Could you check a few things on this drawing? It's one solid part, dimensions in mm from its lowest x, y, z. Give positions to 0.01 mm unless a question says otherwise; leave off trailing zeros. Loops run counter-clockwise (first coordinate to the right, second up) from the corner with the lowest first, then second, coordinate; pieces in that order, holes last. Notation, with made-up numbers: (-10.5, 13) -> (18.5, 13) arc R30 cw to (18.5, 44) -> close; hole circle Ø6 at (85.5, 53.5). An arc over 180 degrees is marked (long way). Use CSV: the item, a comma, the result in double quotes.
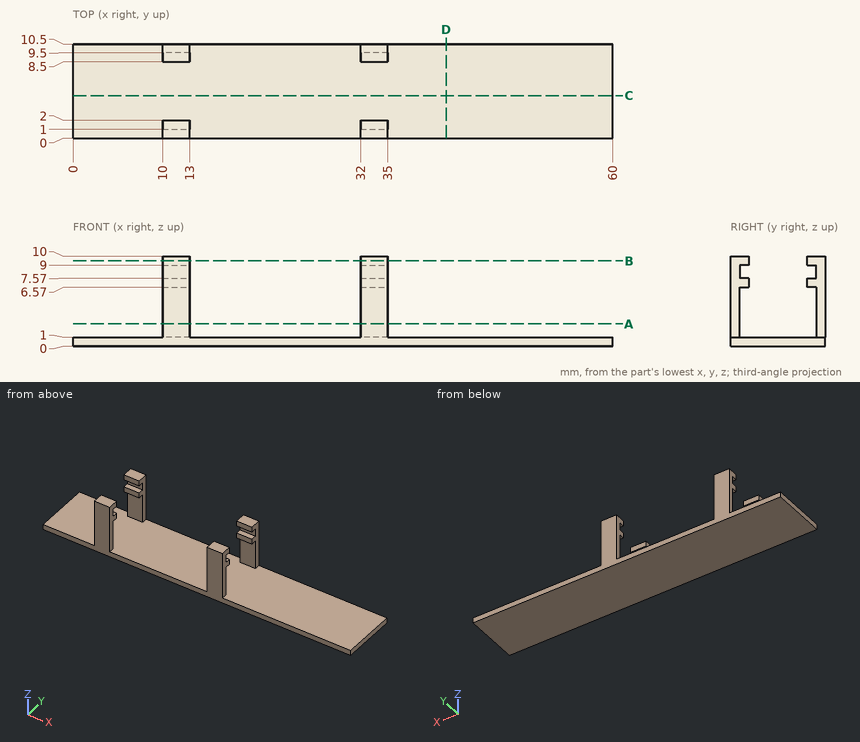
(1) If I drill on L1, parallel to X at y = 9.75, z = 7; L2, parallel to Z at x = 10.5, y = 7.25, over which ranges is the centre line in solid material (lowest first)? Write a range as from..to.
Answer sheet:
L1,"x = 10..13, 32..35"
L2,"z = 0..1"
(2) If we section it at A-A, the plane z = 2.5: Write out the boundary of the cut face in (x, y), then the cut area to 3 significant figures.
Answer sheet:
outline,"(10, 0) -> (13, 0) -> (13, 1) -> (10, 1) -> close; (10, 9.5) -> (13, 9.5) -> (13, 10.5) -> (10, 10.5) -> close; (32, 0) -> (35, 0) -> (35, 1) -> (32, 1) -> close; (32, 9.5) -> (35, 9.5) -> (35, 10.5) -> (32, 10.5) -> close"
area,"12.0 mm2"
(3) If we section it at C-C, the plane y = 4.75: Write out the boundary of the cut face in (x, z).
Answer sheet:
outline,"(0, 0) -> (60, 0) -> (60, 1) -> (0, 1) -> close"
(4) If we section it at B-B, the plane z = 9.5: Write out the boundary of the cut face in (x, y), then the cut area to 3 significant figures.
Answer sheet:
outline,"(10, 0) -> (13, 0) -> (13, 2) -> (10, 2) -> close; (10, 8.5) -> (13, 8.5) -> (13, 10.5) -> (10, 10.5) -> close; (32, 0) -> (35, 0) -> (35, 2) -> (32, 2) -> close; (32, 8.5) -> (35, 8.5) -> (35, 10.5) -> (32, 10.5) -> close"
area,"24.0 mm2"
(5) If we section it at D-D, the plane x = 41.5: Write out the boundary of the cut face in (y, z).
Answer sheet:
outline,"(0, 0) -> (10.5, 0) -> (10.5, 1) -> (0, 1) -> close"
(6) Will these pins go through, and if not, where does the flat tip stop? pin 1 Ø1 at (y, z) = (9.5, 6) entering from -X; pin 2 Ø3 at (x, y) = (46.5, 3) entering from +Z; pin 3 Ø2 at (y, z) = (9.5, 3.5) entering from +X.
Answer sheet:
pin 1,"stops at x = 10"
pin 2,"stops at z = 1"
pin 3,"stops at x = 35"
